The listing builds one solid part. Answer for the finished solid, in the listing's coordinates (mm). A direction names the side the tool comes from. Give positions to 0.01 mm unless a question says otherwise; leave off trailing zeros. Write each loop counter-clockwise with the first axis right and the second up, starting at its lowest first coordinate (ties: lowest second). Pieces come first, ordered by that corner, then holes. Notation, with made-up numbers: M 38,86 L 53,86 A25 cw 53,106 Z; hole C 2,-38.5 d6. An arc over 180 degrees is marked long. Return JSON: item names as keys, results as strings.
from build123d import *

# Parameters (mm, degrees)
SKETCH1_R           = 45.339
BOSS_EXTRUDE2_DEPTH = 38.1
SKETCH3_R           = 41.529
CUT_EXTRUDE1_DEPTH  = 50.8
SKETCH4_R           = 20.0025
CUT_EXTRUDE2_DEPTH  = 25.4
CHAMFER1_SIZE       = 10


with BuildPart() as part:
    # Sketch1 → Boss-Extrude2 (new, symmetric)
    with BuildSketch(Plane(origin=(0, 0, 0), x_dir=(0, 1, 0), z_dir=(0, 0, 1))):
        with Locations(Location((0, 0, 0), (0, 0, 90))):
            Circle(SKETCH1_R)
    extrude(amount=BOSS_EXTRUDE2_DEPTH, both=True)

    # Sketch3 → Cut-Extrude1 (cut)
    with BuildSketch(Plane.XY.offset(38.1)):
        Circle(SKETCH3_R)
    extrude(amount=-CUT_EXTRUDE1_DEPTH, mode=Mode.SUBTRACT)

    # Sketch4 → Cut-Extrude2 (cut)
    with BuildSketch(Plane(origin=(0, 0, -38.1), x_dir=(1, 0, 0), z_dir=(0, 0, -1))):
        with Locations(Location((0, 0, 0), (0, 0, 180))):
            Circle(SKETCH4_R)
    extrude(amount=-CUT_EXTRUDE2_DEPTH, mode=Mode.SUBTRACT)

    # Chamfer1
    chamfer1_edges = [part.edges().sort_by_distance(p)[0] for p in [
        (20.0025, 0, -12.7),
        (-41.529, 0, -12.7),
    ]]
    chamfer(chamfer1_edges, length=CHAMFER1_SIZE)


solid = part.part
Item 1: Find the intervals of material crossed by line 1 (Y direction, x = 0, z = 29); line 2 (Y direction, x = 15.5, z = 21.5); line 3 (X direction, y = 10, z = -20.5), in increasing order.
Geometry results:
{"line 1": "y = -45.34 to -41.53, 41.53 to 45.34", "line 2": "y = -42.61 to -38.53, 38.53 to 42.61", "line 3": "x = -44.22 to -19.82, 19.82 to 44.22"}
Item 2: A cutting plane is placed at D-D, the plane z = -33. Write down the section's boundary in (x, y) (1 decimal).
Geometry results:
{"outline": "C 0,0 d90.7; hole C 0,0 d40"}
Item 3: Determine the mould class of faces 3 (the cylindrical face through (-20.921, 40.223, 0.533)), 4 (the conical face through (2.685, 20.453, -22.074)), 5 (the flat face through (-20, 9, -38.1)) for opening direction X: +X half, -X half, draft (parallel to the pull), parting line (faces both ways), or undercut.
Geometry results:
{"face 3": "parting line", "face 4": "undercut", "face 5": "draft"}
Item 4: Given pin 1 Ø10 at (x, z) = (-35, -25.5) entering from -Y; pin 2 Ø5 at (x, z) = (6, -23) entering from -Y; pin 3 Ø1 at (x, z) = (-22.5, -14) entering from +Y, each flat-ended and moving along its own axis, determine where each tip first touches the part or whether it passes through.
Geometry results:
{"pin 1": "stops at y = -33.99", "pin 2": "stops at y = -45.2", "pin 3": "stops at y = 39.64"}
Item 5: Which of the six approach directions +Z, -Z, +X, -X, +Y, -Y give full straight-line access (tool end or side, diameter ignored) to faces 1 (the flat face through (28, -12, -12.7)), 2 (the flat face through (-37, 20, 38.1))?
Geometry results:
{"face 1": "+Z", "face 2": "+Z, +X, -X, +Y, -Y"}
Item 6: A cutting plane is placed at C-C, the plane z = 20. Write down the section's boundary in (x, y), plus the area to 3 significant figures.
Geometry results:
{"outline": "C 0,0 d90.68; hole C 0,0 d83.06", "area": "1,040 mm2"}
Item 7: A cutting plane is placed at A-A, the plane x = 0. Write down the section's boundary in (y, z).
Geometry results:
{"outline": "M -45.34,-38.1 L -20,-38.1 L -20,-22.7 L -30,-12.7 L -31.53,-12.7 L -41.53,-2.7 L -41.53,38.1 L -45.34,38.1 Z; M 20,-38.1 L 45.34,-38.1 L 45.34,38.1 L 41.53,38.1 L 41.53,-2.7 L 31.53,-12.7 L 30,-12.7 L 20,-22.7 Z"}
